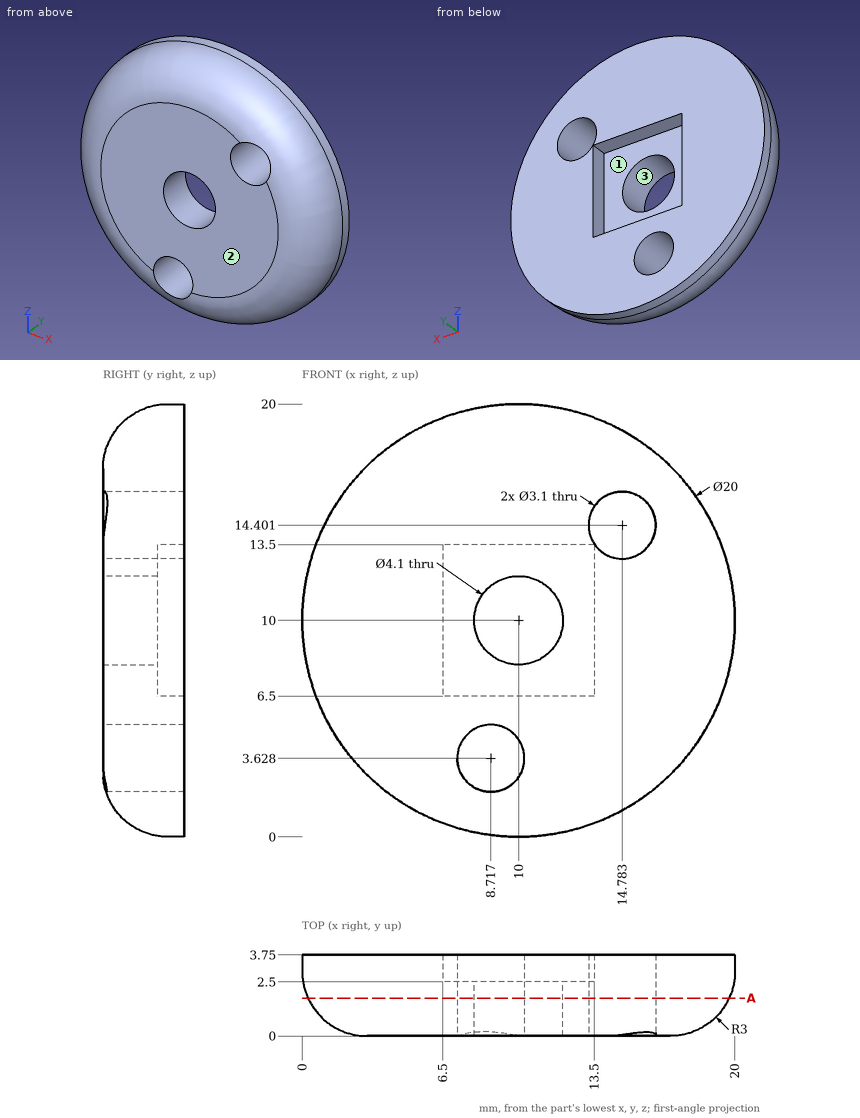
Answer from the drawing. Dimensions are ordinates in mm from the lowest x, y and z of the part. Give positions to 0.01 mm unless a question says otherwise; leave off trailing zeros. One line per item, written item: value. Start each with the question number.
1) Find the intervals of material crossed by L1, parallel to X at y = 2.45, z = 5 (1 decimal); L2, parallel to Z at x = 12.5, y = 2.55; L3, parallel to Z at x = 13.5, y = 1.4 (1 decimal), in increasing order.
2) Given pin 1 Ø0.6 at (y, z) = (3.5, 11) entering from -X (1 decimal); pin 2 Ø1.5 at (x, y) = (4.5, 2) entering from +Z; pin 3 Ø1.5 at (y, z) = (1.5, 5) entering from +X; pin 4 Ø5 at (x, z) = (8.72, 3.63) entering from +Y, each flat-ended and moving along its own axis, determine where each tip first touches the part or whether it passes through.
3) A cutting plane is placed at A-A on y = 1.75. State how many separate pieces and enclosed holes the cut face has, then the cut area to 3 significant figures.
4) The mould has two halves that part along Z. Classify the marked faces 1, 2 and 3: released by +Z, released by -Z, zero draft, split by the parting line, or undercut.
Answer sheet:
1. L1: x = 1.4 to 8, 9.4 to 18.6
1. L2: z = 0.35 to 6.5, 13.5 to 19.65
1. L3: z = 1.1 to 13.5, 15.3 to 18.9
2. pin 1: stops at x = 0
2. pin 2: stops at z = 18.67
2. pin 3: stops at x = 18.77
2. pin 4: stops at y = 3.75
3. separate pieces: 1
3. enclosed holes: 3
3. area: 269 mm2
4. face 1: undercut
4. face 2: zero draft
4. face 3: undercut
